from build123d import *

# Parameters (mm, degrees)
CYLINDER_R     = 0.5
CYLINDER_DEPTH = 16
BOX_W          = 20
BOX_H          = 40
BOX_DEPTH      = 10


with BuildPart() as esfera:
    # Sphere → Sphere (revolve)
    with BuildSketch(Plane(origin=(4, 4, 10), x_dir=(1, 0, 0), z_dir=(0, -1, 0))):
        with BuildLine():
            ThreePointArc((0, -2), (2, 0), (0, 2))
            Line((0, 2), (0, -2))
        make_face()
    revolve(axis=Axis((4, 4, 10), (0, 0, 1)))


with BuildPart() as esfera001:
    # Sphere001 → Sphere001 (revolve)
    with BuildSketch(Plane(origin=(16, 4, 10), x_dir=(1, 0, 0), z_dir=(0, -1, 0))):
        with BuildLine():
            ThreePointArc((0, -2), (2, 0), (0, 2))
            Line((0, 2), (0, -2))
        make_face()
    revolve(axis=Axis((16, 4, 10), (0, 0, 1)))


with BuildPart() as esfera002:
    # Sphere002 → Sphere002 (revolve)
    with BuildSketch(Plane(origin=(10, 10, 10), x_dir=(1, 0, 0), z_dir=(0, -1, 0))):
        with BuildLine():
            ThreePointArc((0, -2), (2, 0), (0, 2))
            Line((0, 2), (0, -2))
        make_face()
    revolve(axis=Axis((10, 10, 10), (0, 0, 1)))


with BuildPart() as esfera003:
    # Sphere003 → Sphere003 (revolve)
    with BuildSketch(Plane(origin=(4, 16, 10), x_dir=(1, 0, 0), z_dir=(0, -1, 0))):
        with BuildLine():
            ThreePointArc((0, -2), (2, 0), (0, 2))
            Line((0, 2), (0, -2))
        make_face()
    revolve(axis=Axis((4, 16, 10), (0, 0, 1)))


with BuildPart() as esfera004:
    # Sphere004 → Sphere004 (revolve)
    with BuildSketch(Plane(origin=(16, 16, 10), x_dir=(1, 0, 0), z_dir=(0, -1, 0))):
        with BuildLine():
            ThreePointArc((0, -2), (2, 0), (0, 2))
            Line((0, 2), (0, -2))
        make_face()
    revolve(axis=Axis((16, 16, 10), (0, 0, 1)))


with BuildPart() as cilindre:
    # Cylinder → Cylinder (new body)
    with BuildSketch(Plane(origin=(2, 20, 10), x_dir=(0, 0, -1), z_dir=(1, 0, 0))):
        Circle(CYLINDER_R)
    extrude(amount=CYLINDER_DEPTH)


with BuildPart() as esfera007:
    # Sphere007 → Sphere007 (revolve)
    with BuildSketch(Plane(origin=(16, 24, 10), x_dir=(1, 0, 0), z_dir=(0, -1, 0))):
        with BuildLine():
            ThreePointArc((0, -2), (2, 0), (0, 2))
            Line((0, 2), (0, -2))
        make_face()
    revolve(axis=Axis((16, 24, 10), (0, 0, 1)))


with BuildPart() as esfera006:
    # Sphere006 → Sphere006 (revolve)
    with BuildSketch(Plane(origin=(10, 30, 10), x_dir=(1, 0, 0), z_dir=(0, -1, 0))):
        with BuildLine():
            ThreePointArc((0, -2), (2, 0), (0, 2))
            Line((0, 2), (0, -2))
        make_face()
    revolve(axis=Axis((10, 30, 10), (0, 0, 1)))


with BuildPart() as esfera005:
    # Sphere005 → Sphere005 (revolve)
    with BuildSketch(Plane(origin=(4, 36, 10), x_dir=(1, 0, 0), z_dir=(0, -1, 0))):
        with BuildLine():
            ThreePointArc((0, -2), (2, 0), (0, 2))
            Line((0, 2), (0, -2))
        make_face()
    revolve(axis=Axis((4, 36, 10), (0, 0, 1)))


with BuildPart() as cut008:
    # Box → Box (new body)
    with BuildSketch(Plane.XY):
        with Locations((10, 20)):
            Rectangle(BOX_W, BOX_H)
    extrude(amount=BOX_DEPTH)

    # Cut: cut Esfera005
    add(esfera005.part, mode=Mode.SUBTRACT)

    # Cut001: cut Esfera006
    add(esfera006.part, mode=Mode.SUBTRACT)

    # Cut002: cut Esfera007
    add(esfera007.part, mode=Mode.SUBTRACT)

    # Cut003: cut Cilindre
    add(cilindre.part, mode=Mode.SUBTRACT)

    # Cut004: cut Esfera004
    add(esfera004.part, mode=Mode.SUBTRACT)

    # Cut005: cut Esfera003
    add(esfera003.part, mode=Mode.SUBTRACT)

    # Cut006: cut Esfera002
    add(esfera002.part, mode=Mode.SUBTRACT)

    # Cut007: cut Esfera001
    add(esfera001.part, mode=Mode.SUBTRACT)

    # Cut008: cut Esfera
    add(esfera.part, mode=Mode.SUBTRACT)


solid = cut008.part
Here's how the part is built. I have some questions about the finished solid (model axes, mm). Round coordinates to 2 decimals unless told otherwise and drop trailing zeros. Loops run counter-clockwise (first coordinate to the right, second up) from the corner with the lowest first, then second, coordinate; pieces in that order, holes last. Notation, with made-up numbers: (-39, 2) - (-34, 2) arc R34 cw to (-34, 39) - close; hole circle Ø4 at (-6, -22.75). An arc over 180 degrees is marked (long way). One line per question, with ' | ' between items. Start each with the question number.
Q1. Will this pin go through, and if not, where does the flat tip stop? pin 1 (1 mm diameter, centred on x = 12.5, y = 21.5, fed in from -Z).
Q2. I want a section at C-C (x = 14.5). Write out the boundary of the cut face in (y, z).
Q3. I want a section at A-A (y = 20). Write out the boundary of the cut face in (x, z), then the cut area to 3 significant figures.
Q4. I want a section at B-B (x = 8.75). Write out the boundary of the cut face in (y, z).
Q5. I want a section at D-D (y = 9.5). Write out the boundary of the cut face in (x, z).
Q6. Please list where these lines run through material, in increasing order: line 1 (Y direction, x = 2.75, z = 9.75); line 2 (Z direction, x = 15.5, y = 23.5). Write a range as [from, to].
Q7. We'd pull the mould along Y, two halves only. Please class faces 1 (the cylindrical face through (9.9, 20, 9.5)), 2 (the flat face through (20, 20, 5)), 3 (the flat face through (10, 0, 5)): +Y half, -Y half, draft (parallel to the pull), parting line (faces both ways), or undercut.
Response values:
1) pin 1: stops at z = 0
2) outline: (0, 0) - (40, 0) - (40, 10) - (25.32, 10) arc R1.32 cw to (22.68, 10) - (20.5, 10) arc R0.5 cw to (19.5, 10) - (17.32, 10) arc R1.32 cw to (14.68, 10) - (5.32, 10) arc R1.32 cw to (2.68, 10) - (0, 10) - close
3) outline: (0, 0) - (20, 0) - (20, 10) - (18, 10) - (18, 9.5) - (2, 9.5) - (2, 10) - (0, 10) - close | area: 192 mm²
4) outline: (0, 0) - (40, 0) - (40, 10) - (31.56, 10) arc R1.56 cw to (28.44, 10) - (20.5, 10) arc R0.5 cw to (19.5, 10) - (11.56, 10) arc R1.56 cw to (8.44, 10) - (0, 10) - close
5) outline: (0, 0) - (20, 0) - (20, 10) - (11.94, 10) arc R1.94 cw to (8.06, 10) - (0, 10) - close
6) line 1: y = [0, 2.46], [5.54, 14.46], [17.54, 19.57], [20.43, 34.46], [37.54, 40] | line 2: z = [0, 8.13]
7) face 1: undercut | face 2: draft | face 3: -Y half
